The drawing under review shows one solid part. Ordinate dimensions are in mm from its lowest x, y, z. Coordinates: 2 decimals unless noted, no trailing zeros. Order: outer loops, then holes, each group sorted by start corner. A loop starts at its lowest first (then second) coordinate and runs counter-clockwise, first axis right, second up. Notation, with made-up numbers: (32, 11.5) -> (59, 11.5) arc R14 ccw to (59, 34.5) -> close; hole circle Ø3 at (7.25, -37.5). An arc over 180 degrees is marked (long way). Put each result on its own line as item: value.
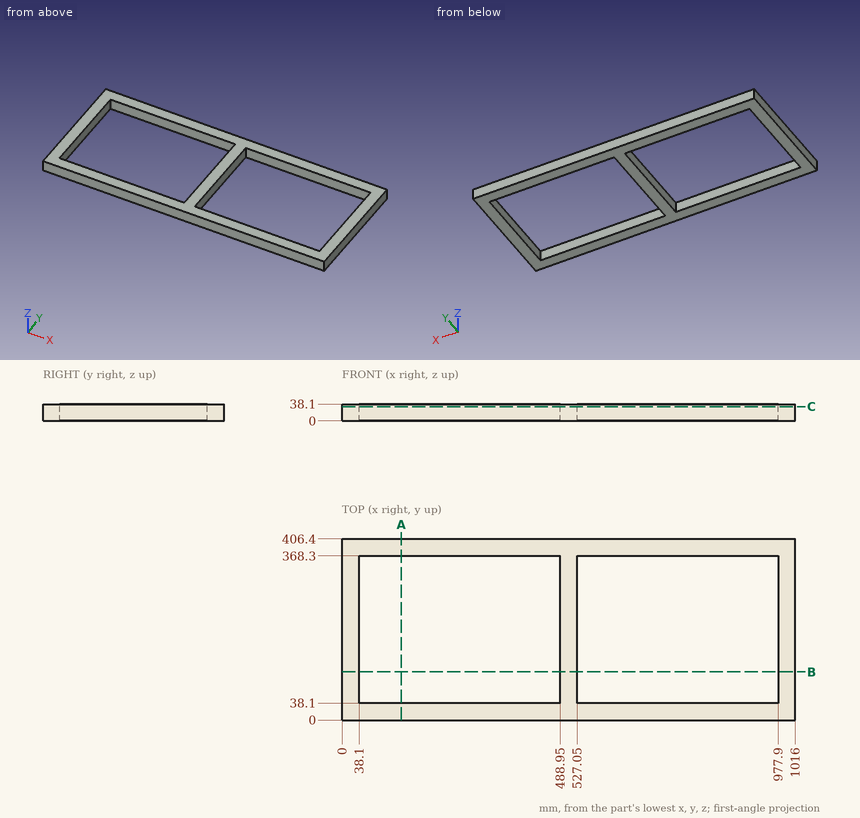
Item 1: Consider section B-B on y = 108.5. Write out the cut boundary in (x, z), and give its area (3 significant figures).
Answers below:
outline: (0, 0) -> (38.1, 0) -> (38.1, 38.1) -> (0, 38.1) -> close; (488.95, 0) -> (527.05, 0) -> (527.05, 38.1) -> (488.95, 38.1) -> close; (977.9, 0) -> (1016, 0) -> (1016, 38.1) -> (977.9, 38.1) -> close
area: 4,350 mm^2
Item 2: Consider section C-C on z = 32. Write out the cut boundary in (x, y), and give its area (3 significant figures).
Answers below:
outline: (0, 0) -> (1016, 0) -> (1016, 406.4) -> (0, 406.4) -> close; hole (38.1, 38.1) -> (488.95, 38.1) -> (488.95, 368.3) -> (38.1, 368.3) -> close; hole (527.05, 38.1) -> (977.9, 38.1) -> (977.9, 368.3) -> (527.05, 368.3) -> close
area: 115,000 mm^2
Item 3: For line 1 (X direction, y = 314, z = 9); line 2 (Y direction, x = 118, z = 24), list the stretches that pass through material, from the lowest coordinate up. Write a range as from..to.
Answers below:
line 1: 0..38.1, 488.95..527.05, 977.9..1016
line 2: 0..38.1, 368.3..406.4
Item 4: Consider section A-A on x = 133. Write out the cut boundary in (y, z), and give its area (3 significant figures).
Answers below:
outline: (0, 0) -> (38.1, 0) -> (38.1, 38.1) -> (0, 38.1) -> close; (368.3, 0) -> (406.4, 0) -> (406.4, 38.1) -> (368.3, 38.1) -> close
area: 2,900 mm^2
